Geometry: see drawing. Coordinates: mm, zero at the bounding-box minimum. A direction names the side the tool comes from. Coordinates: 2 decimals unless noted, no trailing zeros. Write each loop counter-clockwise with the first axis right and the second up, starting at its lowest first coordinate (ties: lowest second). Pieces come first, ordered by that corner, then holes. Notation, with made-up numbers: (-25, -21.5) - (13, -21.5) arc R19 cw to (13, -1.5) - close; hole circle Ø3 at (6.5, 81.25). An arc over 180 degrees is marked (long way). Use a Markdown table: item, result. Add a question column.
Q1. Section query C-C (x = 9). Return the cut outline in (y, z).
Q2. Material intervals for probe 1 along Y at (x, z) = (13, 22.5); probe 2 along Z at (x, y) = (15, 1.1), sorted ascending. Write a range as from..to.
Q3. Section query D-D (z = 20). Return the cut outline in (x, y).
Q4. Mould query, pull axis X, two halves, no side actions, for the marked faces 1, 2 and 3. Classes: released by +X, released by -X, zero draft, split by the parting line, or undercut.
Q5. Pin query (flat end, axial travel): P1, Ø12, axis at x = 21, y = 13.5, coming from the +Z side; P2, Ø9, axis at x = 23.5, z = 16.5, coming from the +Y side; P3, Ø2.5, axis at x = 15.5, y = 16.5, coming from the +Z side. Return the tip coordinate at first contact, or that it passes through.
Q6. Set-up query: the marked faces 4 and 5. Return all of +Z, -Z, +X, -X, +Y, -Y with unobstructed straight access to the full face (end or side cutting, diameter ignored); none if empty.
Q7. Section query A-A (y = 4.5). Return the cut outline in (x, z).
Q8. Section query B-B (y = 15). Return the cut outline in (x, z) (1 decimal).
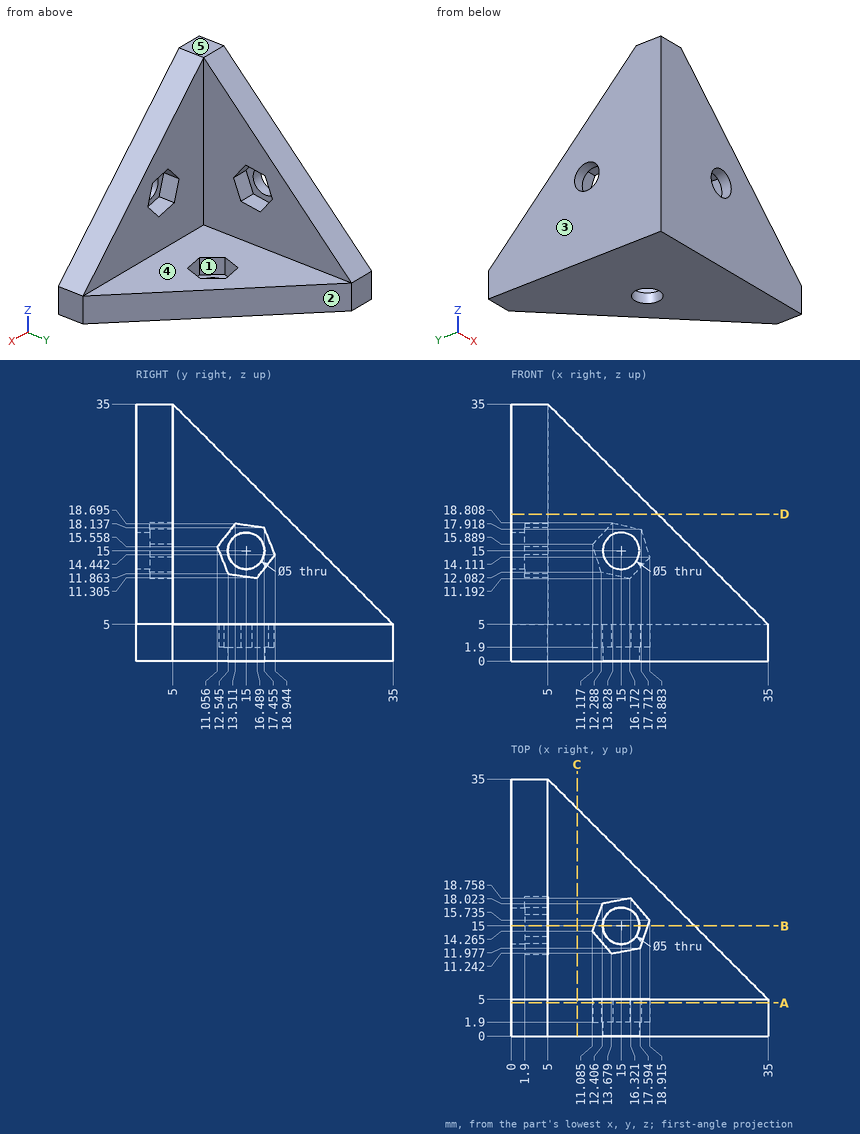
Values follow:
| question | item | result |
|---|---|---|
| 1 | outline | (0, 0) - (31, 0) - (31, 5) - (5, 5) - (5, 31) - (0, 31) - close |
| 2 | probe 1 | 0..5 |
| 2 | probe 2 | 0..12.5, 17.5..25 |
| 3 | outline | (0, 0) - (20, 0) - (20, 5) - (5, 5) - (5, 20) - (0, 20) - close |
| 4 | face 1 | undercut |
| 4 | face 2 | released by +X |
| 4 | face 3 | released by -X |
| 5 | P1 | z = 5 |
| 5 | P2 | y = 5 |
| 5 | P3 | z = 1.9 |
| 6 | face 4 | +Z, +X, +Y |
| 6 | face 5 | +Z, +X, -X, +Y, -Y |
| 7 | outline | (0, 0) - (35, 0) - (35, 5) - (5, 35) - (0, 35) - close; hole (11.12, 15.89) - (12.29, 12.08) - (16.17, 11.19) - (18.88, 14.11) - (17.71, 17.92) - (13.83, 18.81) - close |
| 8 | outline | (0, 0) - (12.5, 0) - (12.5, 1.9) - (11.3, 1.9) - (11.3, 5) - (5, 5) - (5, 11.5) - (1.9, 11.5) - (1.9, 12.5) - (0, 12.5) - close; (0, 17.5) - (1.9, 17.5) - (1.9, 18.5) - (5, 18.5) - (5, 25) - (0, 25) - close; (17.5, 0) - (25, 0) - (25, 5) - (18.7, 5) - (18.7, 1.9) - (17.5, 1.9) - close |
